Answer from the drawing. Dimensions are ordinates in mm from the lowest x, y and z of the part. Coordinates: 2 decimals unless noted, no trailing zeros. Loops run counter-clockwise (first coordinate to the right, second up) from the corner with the lowest first, then second, coordinate; pieces in that order, holes last. Notation, with made-up numbers: (75.5, -40) -> (118.5, -40) arc R30 cw to (118.5, -15) -> close; hole circle Ø10 at (4, 26.5). An arc over 180 degrees is marked (long way). Answer as CSV lines item,"result".
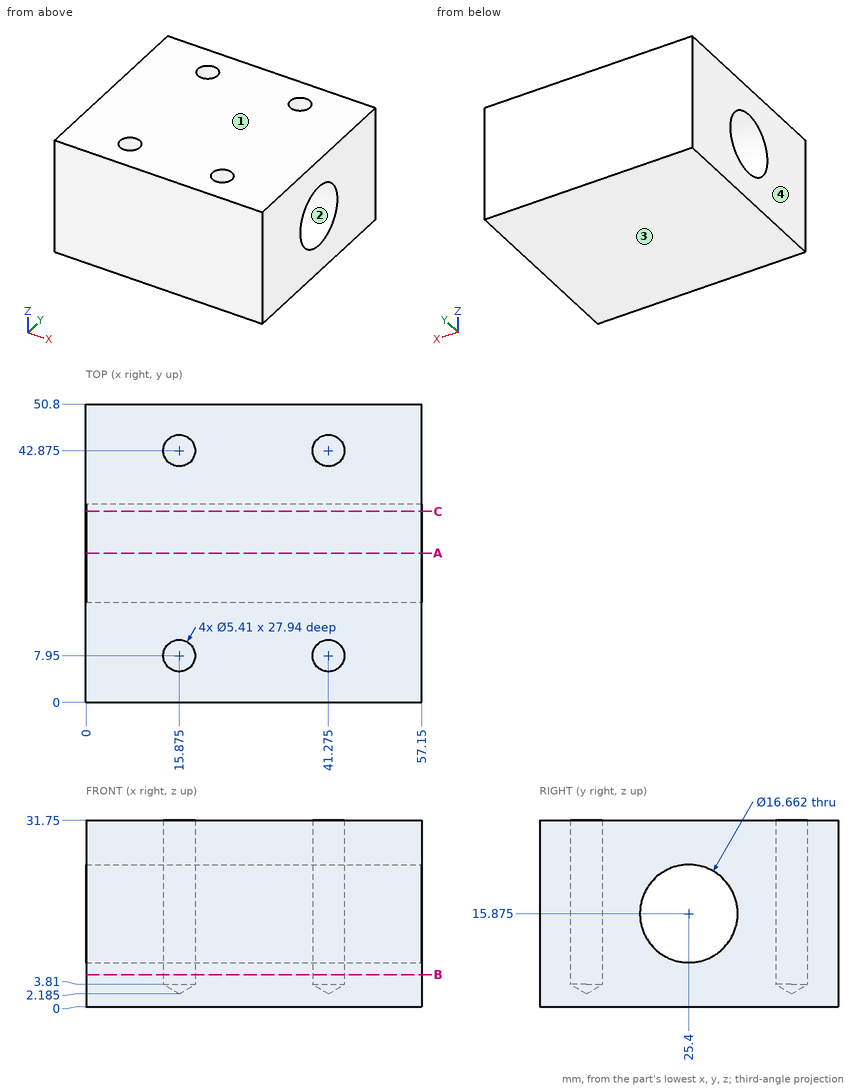
(1) For a pull along Z with two mould halves and no side action, classify the marked faces 1, 2, 3 and 4 as pulls with the +Z half, pulls with the -Z half, needs draft (parallel to the pull), parting line crosses it, or undercut.
Computed values:
face 1,"pulls with the +Z half"
face 2,"undercut"
face 3,"pulls with the -Z half"
face 4,"needs draft"
(2) A cutting plane is placed at A-A, the plane y = 25.4. Write down the section's boundary in (x, z), and give its area (3 significant figures).
Computed values:
outline,"(0, 0) -> (57.15, 0) -> (57.15, 7.54) -> (0, 7.54) -> close; (0, 24.21) -> (57.15, 24.21) -> (57.15, 31.75) -> (0, 31.75) -> close"
area,"862 mm2"
(3) A cutting plane is placed at B-B, the plane z = 5.5. Count the separate pieces of the cut face and the enclosed holes in it, and give its area (3 significant figures).
Computed values:
separate pieces,"1"
enclosed holes,"4"
area,"2,810 mm2"
(4) A flat-ended cylindrical pin translates along its axis: pin 1 Ø3 at (x, y) = (15.88, 7.95) entering from +Z. Find the tip coordinate at first contact, or state that the pin passes through.
Computed values:
pin 1,"z = 3.09"
(5) A cutting plane is placed at C-C, the plane y = 32.5. Write down the section's boundary in (x, z).
Computed values:
outline,"(0, 0) -> (57.15, 0) -> (57.15, 11.52) -> (0, 11.52) -> close; (0, 20.23) -> (57.15, 20.23) -> (57.15, 31.75) -> (0, 31.75) -> close"
(6) Consider line 1 along X through (y, z) = (8, 11); line 2 along Y through (x, z) = (52, 15.5); line 3 along Y through (x, z) = (41, 13.5) (1 decimal). Determine where each line is inside the solid, lowest interval first.
Computed values:
line 1,"0 to 13.17, 18.58 to 38.57, 43.98 to 57.15"
line 2,"0 to 17.08, 33.72 to 50.8"
line 3,"0 to 5.3, 10.6 to 17.4, 33.4 to 40.2, 45.6 to 50.8"
